Build history of the part. All positions in model axes, mm. Round coordinates to 2 decimals unless told otherwise and drop trailing zeros. Order: outer loops, then holes, each group sorted by start corner. A loop starts at its lowest first (then second) coordinate and runs counter-clockwise, first axis right, second up. Notation, with made-up numbers: (6.25, 13) -> (51.25, 13) arc R11 cw to (51.25, 18) -> close; hole circle Ø8 at (53, -17.75). An arc over 180 degrees is marked (long way). Answer as a JSON object with one key per item and string values.
Autodesk Inventor part; units mm, degrees
ref_plane "YZ Plane" through (0, 0, 0) normal (1, 0, 0) x (0, 1, 0)
ref_plane "XZ Plane" through (0, 0, 0) normal (0, 1, 0) x (-1, 0, 0)
ref_plane "XY Plane" through (0, 0, 0) normal (0, 0, 1) x (1, 0, 0)
sketch "Sketch1" plane through (0, 0, 0) normal (0, 0, 1) x (1, 0, 0)
  line L0 (-4, 2.75) -> (-7, 2.75)
  line L1 (-7, 2.75) -> (-7, -2.75)
  line L2 (-7, -2.75) -> (7, -2.75)
  line L3 (7, -2.75) -> (7, 2.75)
  line L4 (7, 2.75) -> (4, 2.75)
  line L5 (4, 2.75) -> (5, 0.75)
  line L6 (5, 0.75) -> (-5, 0.75)
  line L7 (-5, 0.75) -> (-4, 2.75)
  point P0 (0, 0)
  point P1 (0, 0.75)
  point P2 (0, -2.75)
  point P3 (-7, 0)
  dimension "d0" = 14
  dimension "d2" = 3.5
  dimension "d4" = 10
  dimension "d19" = 5.5
  dimension "d20" = 8
extrude "Extrusion1" add sketch "Sketch1" against normal mid plane 170
sketch "Sketch2" plane through (-7, -2.75, -85) normal (0, -1, 0) x (1, 0, 0)
  circle A0 centre (7, 165) radius 1.6
  circle A1 centre (7, 135) radius 1.6
  circle A2 centre (7, 105) radius 1.6
  circle A3 centre (7, 70) radius 1.6
  circle A4 centre (7, 40) radius 1.6
  circle A5 centre (7, 10) radius 1.6
  point P0 (7, 85)
  dimension "d7" = 3.2
  dimension "d8" = 15
  dimension "d9" = 20
  dimension "d10" = 30
  dimension "d11" = 30
  dimension "d12" = 30
  dimension "d13" = 30
extrude "Extrusion2" cut sketch "Sketch2" against normal through all
sketch "Sketch3" plane through (-5, 0.75, -85) normal (0, 1, 0) x (1, 0, 0)
  circle A0 centre (5, -165) radius 1.6
  circle A1 centre (5, -135) radius 1.6
  circle A2 centre (5, -135) radius 1.6
  circle A3 centre (5, -105) radius 1.6
  circle A4 centre (5, -105) radius 1.6
  circle A5 centre (5, -70) radius 1.6
  circle A6 centre (5, -40) radius 1.6
  circle A7 centre (5, -10) radius 1.6
  circle A8 centre (5, -165) radius 3
  circle A9 centre (5, -135) radius 3
  circle A10 centre (5, -105) radius 1.6
  circle A11 centre (5, -105) radius 3
  circle A12 centre (5, -70) radius 1.6
  circle A13 centre (5, -70) radius 3
  circle A14 centre (5, -40) radius 3
  circle A15 centre (5, -10) radius 1.6
  circle A16 centre (5, -10) radius 3
  point P0 (5, -85)
  dimension "d16" = 6
extrude "Extrusion3" cut sketch "Sketch3" against normal blind 2.5 contours A0 | A1 | A3 | A5 | A6 | A7 | A8 | A9 | A11 | A13 | A14 | A16
equation "\"d11\" = d10"
equation "\"d12\" = d10"
equation "\"d13\" = d10"
properties part number "Rail"
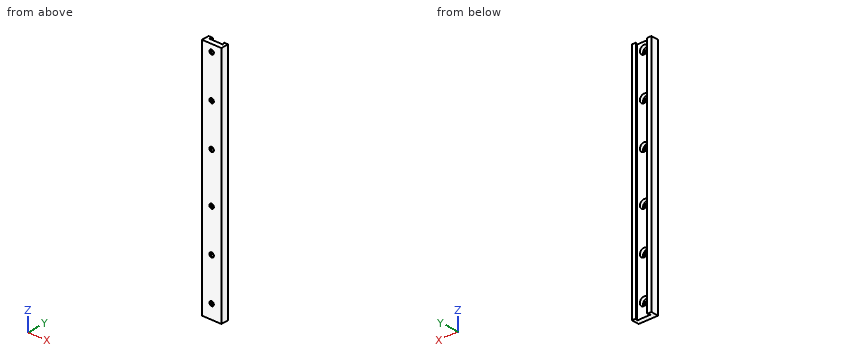
1) Probe L1, parallel to X at y = -0.65, z = -45; L2, parallel to Y at x = -1, z = -71; L3, parallel to X at y = 2.35, z = -51. List the from-to ranges inside material, lowest first. Write a range as from..to.
Checked values:
{"L1": "x = -7..-3, 3..7", "L2": "y = -2.75..0.75", "L3": "x = -7..-4.2, 4.2..7"}
2) Cut at C-C, the plane z = -51. Give the cut face in (x, y).
Checked values:
{"outline": "(-7, -2.75) -> (7, -2.75) -> (7, 2.75) -> (4, 2.75) -> (5, 0.75) -> (-5, 0.75) -> (-4, 2.75) -> (-7, 2.75) -> close"}
3) Cut at D-D, the plane x = 0. Count the separate pieces of the cut face and the enclosed holes in it, plus the area to 3 significant figures.
Checked values:
{"separate pieces": "7", "enclosed holes": "0", "area": "486 mm²"}
4) Cut at B-B, the plane z = 20. Give the cut face in (x, y), plus the area to 3 significant figures.
Checked values:
{"outline": "(-7, -2.75) -> (-1.6, -2.75) -> (-1.6, -1.75) -> (-3, -1.75) -> (-3, 0.75) -> (-5, 0.75) -> (-4, 2.75) -> (-7, 2.75) -> close; (1.6, -2.75) -> (7, -2.75) -> (7, 2.75) -> (4, 2.75) -> (5, 0.75) -> (3, 0.75) -> (3, -1.75) -> (1.6, -1.75) -> close", "area": "40.8 mm²"}
5) Flat gauge pins, fed straight in: pin 1 Ø5.5 at (x, z) = (0, 80) entering from +Y; pin 2 Ø1.9 at (x, z) = (0, -15) entering from -Y. Where does each tip first touch, or does it go through?
Checked values:
{"pin 1": "stops at y = -1.75", "pin 2": "passes through"}
6) Cut at A-A, the plane y = -0.3. Give the cut face in (x, z), plus the area to 3 significant figures.
Checked values:
{"outline": "(-7, -85) -> (7, -85) -> (7, 85) -> (-7, 85) -> close; hole circle Ø6 at (0, -75); hole circle Ø6 at (0, -45); hole circle Ø6 at (0, -15); hole circle Ø6 at (0, 20); hole circle Ø6 at (0, 50); hole circle Ø6 at (0, 80)", "area": "2,210 mm²"}
